from build123d import *

# Parameters (mm, degrees)
SKETCH_1_R      = 1.5
EXTRUDE_1_DEPTH = 25.2


with BuildPart() as part:
    # 草图1 → 凸台-拉伸1 (new body)
    with BuildSketch(Plane.XY):
        with BuildLine():
            ThreePointArc((-13.651838143, 7.126521965), (-14.525683909, 5.115125313), (-15.104966071, 3))
            Line((-15.104966071, 3), (1.6e-08, 3))
            ThreePointArc((1.6e-08, 3), (-7.130933806, 4.054175866), (-13.651838143, 7.126521965))
        make_face()
        with BuildLine():
            Line((1.6e-08, 3), (-15.104966071, 3))
            ThreePointArc((-15.104966071, 3), (-15.326064033, 1.507236297), (-15.4, 0))
            ThreePointArc((-15.4, 0), (-15.326064033, -1.507236297), (-15.104966071, -3))
            Line((-15.104966071, -3), (0, -3))
            Line((0, -3), (15.104966071, -3))
            ThreePointArc((15.104966071, -3), (15.326064033, -1.507236297), (15.4, 0))
            ThreePointArc((15.4, 0), (15.326064033, 1.507236297), (15.104966071, 3))
            Line((15.104966071, 3), (1.6e-08, 3))
        make_face()
        Circle(SKETCH_1_R, mode=Mode.SUBTRACT)
        with BuildLine():
            Line((0, -3), (-15.104966071, -3))
            ThreePointArc((-15.104966071, -3), (-14.525683909, -5.115125313), (-13.651838143, -7.126521965))
            ThreePointArc((-13.651838143, -7.126521965), (-7.130933814, -4.054175868), (0, -3))
        make_face()
        with BuildLine():
            ThreePointArc((13.651838143, 7.126521965), (7.130933821, 4.05417587), (1.6e-08, 3))
            Line((1.6e-08, 3), (15.104966071, 3))
            ThreePointArc((15.104966071, 3), (14.525683909, 5.115125313), (13.651838143, 7.126521965))
        make_face()
        with BuildLine():
            Line((15.104966071, -3), (0, -3))
            ThreePointArc((0, -3), (7.130933814, -4.054175868), (13.651838143, -7.126521965))
            ThreePointArc((13.651838143, -7.126521965), (14.525683909, -5.115125313), (15.104966071, -3))
        make_face()
    extrude(amount=EXTRUDE_1_DEPTH)


solid = part.part
Part model, mm, in its own coordinate system. Round coordinates to 2 decimals unless told otherwise and drop trailing zeros. Loops run counter-clockwise (first coordinate to the right, second up) from the corner with the lowest first, then second, coordinate; pieces in that order, holes last. Notation, with made-up numbers: (-19.75, 10) - (16.25, 10) arc R8 cw to (16.25, 24) - close; hole circle Ø7 at (31, 72). An arc over 180 degrees is marked (long way). Answer as a JSON object with one key per item and string values.
Item 1: Wall check: L1, parallel to X at y = -1, z = 16; L2, parallel to X at y = -0.5, z = 3; L3, parallel to Y at x = 5, z = 18.5. Give the ranges that are in metal, low to high.
Output:
{"L1": "-15.37 to -1.12, 1.12 to 15.37", "L2": "-15.39 to -1.41, 1.41 to 15.39", "L3": "-3.51 to 3.51"}
Item 2: Band-saw the part on A-A on z = 2. List the corners of the cut face in (x, y).
Output:
{"outline": "(-13.65, -7.13) arc R24.65 cw to (13.65, -7.13) arc R15.4 ccw to (13.65, 7.13) arc R24.65 cw to (-13.65, 7.13) arc R15.4 ccw to start; hole circle Ø3 at (0, 0)"}
Item 3: Band-saw the part on B-B on y = -3.5. List the corners of the cut face in (x, z).
Output:
{"outline": "(-15, 0) - (-4.94, 0) - (-4.94, 25.2) - (-15, 25.2) - close; (4.94, 0) - (15, 0) - (15, 25.2) - (4.94, 25.2) - close"}
Item 4: Band-saw the part on C-C on y = -5.25. List the corners of the cut face in (x, z).
Output:
{"outline": "(-14.48, 0) - (-10.29, 0) - (-10.29, 25.2) - (-14.48, 25.2) - close; (10.29, 0) - (14.48, 0) - (14.48, 25.2) - (10.29, 25.2) - close"}
Item 5: Pull direction Y, two halves, no side cores. Call faces 1 (the face through (0, 2, 0)), 2 (the face through (-1.5, 0.07, 12.42)): pulls with the +Y half, pulls with the -Y half, needs draft (parallel to the pull), parting line crosses it, or undercut.
Output:
{"face 1": "needs draft", "face 2": "undercut"}
Item 6: Pin check, flat tips, straight feed: pin 1 (4 mm diameter, centred on y = -4, z = 6, fed in from +X); pin 2 (3 mm diameter, centred on x = -3.5, z = 15, fed in from +Y); pin 3 (2 mm diameter, centred on x = 7, z = 6, fed in from +Y). Stop position of each tip, or through.
Output:
{"pin 1": "x = 15.27", "pin 2": "y = 3.51", "pin 3": "y = 4.33"}
Item 7: Band-saw the part on D-D on x = -9. List the corners of the cut face in (y, z).
Output:
{"outline": "(-4.7, 0) - (4.7, 0) - (4.7, 25.2) - (-4.7, 25.2) - close"}
